Verification items for the finished model (mm, model axes). A direction names the side the tool comes from. Coordinates: 2 decimals unless noted, no trailing zeros. Use one line per item in the form item = value. Start each with the question number.
(1) Mould release check, pull along Z, two halves, no side actions. Record for faces 5 (the cylindrical face through (-68.31, 7.83, 5.85)), 6 (the cylindrical face through (-43.697, 7.985, 0.247)), 7 (the flat face through (-73, 1, 3.25)), 8 (the cylindrical face through (-14.71, 8.87, 8.15)): released by +Z, released by -Z, zero draft, split by the parting line, or undercut.
(2) Tool access check on faces 1 (the cylindrical face through (-52.84, -5.89, 8.75)), 2 (the flat face through (-68.07, 10.307, 4.528)), 3 (the flat face through (-32, 2, 1)), 4 (the flat face through (-66.47, -0.41, 1.6)). Record the directions out of +Z, -Z, +X, -X, +Y, -Y that give a thin tool (end or side, any length) a straight path to the whole face; none if there is none.
(3) Gauge pin test, flat ends, axial feed: pin 1 Ø11 at (x, y) = (-69.5, -2) entering from +Z; pin 2 Ø12 at (x, y) = (1.5, 3) entering from -Z; pin 3 Ø1.5 at (y, z) = (-6.5, 5) entering from +X. Record the tip position at first contact, or that the pin passes through.
(4) Material ranges on line 1 (X direction, y = 0, z = 3.5); line 2 (Y direction, x = 0, z = 3.5); line 3 (Y direction, x = -58, z = 8.75), recorded low to high. Write a range as [from, to].
from build123d import *

# Parameters (mm, degrees)
SKETCH1_R               = 12
SKETCH1_R_2             = 7
BOSS_EXTRUDE1_DEPTH     = 9
SKETCH2_R               = 2
CUT_EXTRUDE1_DEPTH      = 56.352885683
CUT_EXTRUDE1_DEPTH_BACK = 4
CUT_EXTRUDE2_DEPTH      = 8
CUT_EXTRUDE3_DEPTH      = 64.35288577
CUT_EXTRUDE3_DEPTH_BACK = 11.895825623
FILLET1_R               = 1
CUT_EXTRUDE6_DEPTH      = 1
FILLET2_R               = 0.5
FILLET2_OF_MIRROR1_R    = 0.5


with BuildPart() as part:
    # Sketch1 → Boss-Extrude1 (new body)
    with BuildSketch(Plane.XY):
        with BuildLine():
            ThreePointArc((-1.254341216, -11.934262781), (-12, 0), (-1.254341216, 11.934262781))
            Line((-1.254341216, 11.934262781), (-28.139253345, 9.108544651))
            ThreePointArc((-28.139253345, 9.108544651), (-43.686422074, 9.501145293), (-58.610412286, 13.876428933))
            ThreePointArc((-58.610412286, 13.876428933), (-66.906935733, 15.936080839), (-75.412344731, 15.080227428))
            Line((-75.412344731, 15.080227428), (-69.509618943, 4.856406461))
            Line((-69.509618943, 4.856406461), (-62.581415713, 8.856406461))
            Line((-62.581415713, 8.856406461), (-56.581415713, -1.535898385))
            Line((-56.581415713, -1.535898385), (-63.509618943, -5.535898385))
            Line((-63.509618943, -5.535898385), (-61.25902363, -9.434043814))
            ThreePointArc((-61.25902363, -9.434043814), (-53.171617313, -7.441957747), (-44.842954804, -7.352914883))
            Line((-44.842954804, -7.352914883), (-1.254341216, -11.934262781))
        make_face()
        Circle(SKETCH1_R)
        Circle(SKETCH1_R_2, mode=Mode.SUBTRACT)
        with BuildLine():
            Line((-69.509618943, 4.856406461), (-75.412344731, 15.080227428))
            ThreePointArc((-75.412344731, 15.080227428), (-82.336431694, 11.949245255), (-88, 6.882685902))
            Line((-88, 6.882685902), (-86.5, 4.284609691))
            Line((-86.5, 4.284609691), (-81.303847577, 7.284609691))
            Line((-81.303847577, 7.284609691), (-76.107695155, 4.284609691))
            Line((-76.107695155, 4.284609691), (-66.705771366, -12))
            ThreePointArc((-66.705771366, -12), (-64.035889066, -10.603475511), (-61.25902363, -9.434043814))
            Line((-61.25902363, -9.434043814), (-63.509618943, -5.535898385))
            Line((-63.509618943, -5.535898385), (-69.509618943, 4.856406461))
        make_face()
    extrude(amount=BOSS_EXTRUDE1_DEPTH)

    # Sketch2 → Cut-Extrude1 (cut, two sides)
    with BuildSketch(Plane(origin=(-19.480290419, 33.740852752, 0), x_dir=(0.866025404, 0.5, 0), z_dir=(0.5, -0.866025404, 0))) as cut_extrude1_sk:
        with BuildLine():
            Line((-63.768892582, 3.25), (-62.330142082, 3.25))
            ThreePointArc((-62.330142082, 3.25), (-62.768892582, 4.5), (-62.330142082, 5.75))
            Line((-62.330142082, 5.75), (-63.768892582, 5.75))
            Line((-63.768892582, 5.75), (-68.08829873, 5.75))
            Line((-68.08829873, 5.75), (-68.08829873, 3.25))
            Line((-68.08829873, 3.25), (-63.768892582, 3.25))
        make_face()
        with BuildLine():
            Line((-62.330142082, 3.25), (-59.207643082, 3.25))
            ThreePointArc((-59.207643082, 3.25), (-58.881765268, 3.837617557), (-58.768892582, 4.5))
            ThreePointArc((-58.768892582, 4.5), (-58.881765268, 5.162382443), (-59.207643082, 5.75))
            Line((-59.207643082, 5.75), (-62.330142082, 5.75))
            ThreePointArc((-62.330142082, 5.75), (-62.768892582, 4.5), (-62.330142082, 3.25))
        make_face()
        with BuildLine():
            Line((-62.330142082, 5.75), (-59.207643082, 5.75))
            ThreePointArc((-59.207643082, 5.75), (-60.768892582, 6.5), (-62.330142082, 5.75))
        make_face()
        with BuildLine():
            ThreePointArc((-62.330142082, 3.25), (-60.768892582, 2.5), (-59.207643082, 3.25))
            Line((-59.207643082, 3.25), (-62.330142082, 3.25))
        make_face()
        with BuildLine():
            Line((-59.207643082, 3.25), (-57.768892582, 3.25))
            Line((-57.768892582, 3.25), (-57.768892582, 5.75))
            Line((-57.768892582, 5.75), (-59.207643082, 5.75))
            ThreePointArc((-59.207643082, 5.75), (-58.881765268, 5.162382443), (-58.768892582, 4.5))
            ThreePointArc((-58.768892582, 4.5), (-58.881765268, 3.837617557), (-59.207643082, 3.25))
        make_face()
        with Locations((-53.768892582, 4.5)):
            Circle(SKETCH2_R)
    extrude(amount=CUT_EXTRUDE1_DEPTH, mode=Mode.SUBTRACT)
    extrude(cut_extrude1_sk.sketch, amount=-CUT_EXTRUDE1_DEPTH_BACK, mode=Mode.SUBTRACT)

    # Sketch2_4 → Cut-Extrude2 (cut)
    with BuildSketch(Plane(origin=(-19.480290419, 33.740852752, 0), x_dir=(0.866025404, 0.5, 0), z_dir=(0.5, -0.866025404, 0))):
        with BuildLine():
            Line((-63.768892582, 3.25), (-62.330142082, 3.25))
            ThreePointArc((-62.330142082, 3.25), (-62.768892582, 4.5), (-62.330142082, 5.75))
            Line((-62.330142082, 5.75), (-63.768892582, 5.75))
            Line((-63.768892582, 5.75), (-68.08829873, 5.75))
            Line((-68.08829873, 5.75), (-68.08829873, 3.25))
            Line((-68.08829873, 3.25), (-63.768892582, 3.25))
        make_face()
        with BuildLine():
            Line((-62.330142082, 3.25), (-59.207643082, 3.25))
            ThreePointArc((-59.207643082, 3.25), (-58.881765268, 3.837617557), (-58.768892582, 4.5))
            ThreePointArc((-58.768892582, 4.5), (-58.881765268, 5.162382443), (-59.207643082, 5.75))
            Line((-59.207643082, 5.75), (-62.330142082, 5.75))
            ThreePointArc((-62.330142082, 5.75), (-62.768892582, 4.5), (-62.330142082, 3.25))
        make_face()
        with BuildLine():
            Line((-62.330142082, 5.75), (-59.207643082, 5.75))
            ThreePointArc((-59.207643082, 5.75), (-60.768892582, 6.5), (-62.330142082, 5.75))
        make_face()
        with BuildLine():
            ThreePointArc((-62.330142082, 3.25), (-60.768892582, 2.5), (-59.207643082, 3.25))
            Line((-59.207643082, 3.25), (-62.330142082, 3.25))
        make_face()
        with BuildLine():
            Line((-59.207643082, 3.25), (-57.768892582, 3.25))
            Line((-57.768892582, 3.25), (-57.768892582, 5.75))
            Line((-57.768892582, 5.75), (-59.207643082, 5.75))
            ThreePointArc((-59.207643082, 5.75), (-58.881765268, 5.162382443), (-58.768892582, 4.5))
            ThreePointArc((-58.768892582, 4.5), (-58.881765268, 3.837617557), (-59.207643082, 3.25))
        make_face()
    extrude(amount=-CUT_EXTRUDE2_DEPTH, mode=Mode.SUBTRACT)

    # Sketch3 → Cut-Extrude3 (cut, two sides)
    with BuildSketch(Plane(origin=(-23.480290419, 40.669055982, 0), x_dir=(0.866025404, 0.5, 0), z_dir=(0.5, -0.866025404, 0))) as cut_extrude3_sk:
        Polygon((-57.768892582, 9), (-72.768892582, 9), (-72.768892582, 6.5), align=None)
        Polygon((-57.768892582, 0), (-72.768892582, 2.5), (-72.768892582, 0), align=None)
    extrude(amount=CUT_EXTRUDE3_DEPTH, mode=Mode.SUBTRACT)
    extrude(cut_extrude3_sk.sketch, amount=-CUT_EXTRUDE3_DEPTH_BACK, mode=Mode.SUBTRACT)

    # Fillet1
    fillet1_edges = [part.edges().sort_by_distance(p)[0] for p in [
        (-56.581415713, -1.535898385, 4.5),
        (-62.581415713, 8.856406461, 4.5),
    ]]
    fillet(fillet1_edges, radius=FILLET1_R)

    # Sketch5 → Cut-Extrude6 (cut)
    with BuildSketch(Plane.XY.offset(9)):
        with BuildLine():
            Line((-61.460580838, -6.084936491), (-60.58344819, -7.6041748))
            ThreePointArc((-60.58344819, -7.6041748), (-52.728383532, -5.879179053), (-44.686162109, -5.86113204))
            Line((-44.686162109, -5.86113204), (-1.097548864, -10.442479901))
            ThreePointArc((-1.097548864, -10.442479901), (10.5, 0), (-1.097548864, 10.442479901))
            Line((-1.097548864, 10.442479901), (-27.98246065, 7.616761808))
            ThreePointArc((-27.98246065, 7.616761808), (-43.918308598, 8.019177466), (-59.215398565, 12.503843197))
            ThreePointArc((-59.215398565, 12.503843197), (-66.039706904, 14.349674352), (-73.104183378, 14.082374693))
            Line((-73.104183378, 14.082374693), (-68.960580838, 6.905444566))
            Line((-68.960580838, 6.905444566), (-64.197441117, 9.655444566))
            ThreePointArc((-64.197441117, 9.655444566), (-62.300393504, 9.905195622), (-60.782377607, 8.740381057))
            Line((-60.782377607, 8.740381057), (-55.782377607, 0.080127019))
            ThreePointArc((-55.782377607, 0.080127019), (-55.532626551, -1.816920594), (-56.697441117, -3.334936491))
            Line((-56.697441117, -3.334936491), (-61.460580838, -6.084936491))
        make_face()
    cut_extrude6 = extrude(amount=-CUT_EXTRUDE6_DEPTH, mode=Mode.SUBTRACT)

    # Fillet2
    fillet2_edges = [part.edges().sort_by_distance(p)[0] for p in [
        (-59.079010977, -4.709936491, 8),
        (-58.282377607, 4.410254038, 8),
        (-66.579010977, 8.280444566, 8),
        (-71.032382108, 10.49390963, 8),
        (-66.039706904, 14.349674352, 8),
        (-14.540004757, 9.029620855, 8),
        (10.5, 0, 8),
        (-22.891855486, -8.151805971, 8),
        (-61.022014514, -6.844555645, 8),
        (-55.532626551, -1.816920594, 8),
        (-62.300393504, 9.905195622, 8),
        (-43.918308598, 8.019177466, 8),
        (-52.728383532, -5.879179053, 8),
    ]]
    fillet(fillet2_edges, radius=FILLET2_R)

    # Mirror1: Cut-Extrude6 across plane
    add(cut_extrude6.mirror(Plane.XY.offset(4.5)), mode=Mode.SUBTRACT)

    # Fillet2 of Mirror1
    fillet2_of_mirror1_edges = [part.edges().sort_by_distance(p)[0] for p in [
        (-59.079010977, -4.709936491, 1),
        (-58.282377607, 4.410254038, 1),
        (-66.579010977, 8.280444566, 1),
        (-71.032382108, 10.49390963, 1),
        (-66.039706904, 14.349674352, 1),
        (-14.540004757, 9.029620855, 1),
        (10.5, 0, 1),
        (-22.891855486, -8.151805971, 1),
        (-61.022014514, -6.844555645, 1),
        (-55.532626551, -1.816920594, 1),
        (-62.300393504, 9.905195622, 1),
        (-43.918308598, 8.019177466, 1),
        (-52.728383532, -5.879179053, 1),
    ]]
    fillet(fillet2_of_mirror1_edges, radius=FILLET2_OF_MIRROR1_R)


solid = part.part
Answers below:
q1.face_5 = undercut
q1.face_6 = zero draft
q1.face_7 = undercut
q1.face_8 = released by +Z
q2.face_1 = +Z
q2.face_2 = none
q2.face_3 = -Z
q2.face_4 = +Z, -Z
q3.pin_1 = 9
q3.pin_2 = 1
q3.pin_3 = 10.53
q4.line_1 = [-57.47, -7], [7, 12]
q4.line_2 = [-12, -7], [7, 12]
q4.line_3 = [-8.39, -6.84], [-4.09, -2.35], [0.92, 3.92], [11.98, 13.61]
